Verification items for the finished model (mm, model axes). Face numbers are marked on the shaded views. A direction names the side the tool comes from. Round coordinates to 2 decimals unless told otherwise and drop trailing zeros. Write each loop counter-clockwise with the first axis right and the second up, starting at its lowest first coordinate (ties: lowest second). Pieces come first, ordered by that corner, then holes.
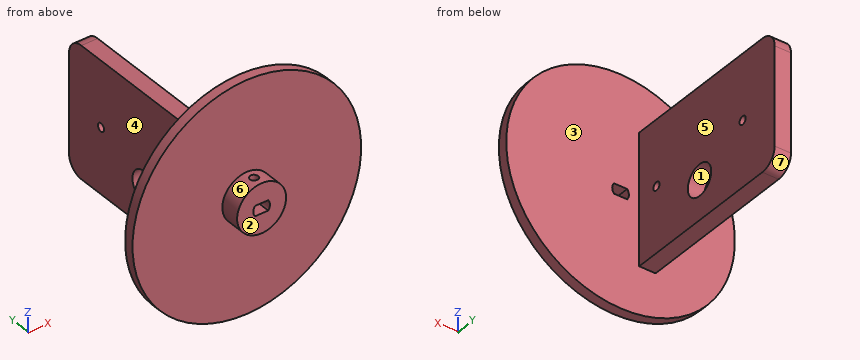
from build123d import *

# Parameters (mm, degrees)
CROQUIS1_R              = 35
SALIENTE_EXTRUIR1_DEPTH = 3
SALIENTE_EXTRUIR2_START = 6
CROQUIS2_R              = 7.5
SALIENTE_EXTRUIR2_DEPTH = 6
CROQUIS3_R              = 1.25
CORTAR_EXTRUIR1_DEPTH   = 6
CROQUIS4_W              = 5
CROQUIS4_H              = 40
SALIENTE_EXTRUIR3_DEPTH = 55
CROQUIS5_R              = 1.25
CROQUIS5_R_2            = 4.75
CORTAR_EXTRUIR2_DEPTH   = 5
REDONDEO1_R             = 5


with BuildPart() as part:
    # Croquis1 → Saliente-Extruir1 (new body)
    with BuildSketch(Plane(origin=(0, 0, 0), x_dir=(1, 0, 0), z_dir=(0, 1, 0))):
        with Locations(Location((0, 0, 0), (0, 0, 270))):
            Circle(CROQUIS1_R)
        with BuildLine():
            Line((-2.024845673, 1.55), (2.024845673, 1.55))
            ThreePointArc((2.024845673, 1.55), (2.55, 0), (2.024845673, -1.55))
            Line((2.024845673, -1.55), (-2.024845673, -1.55))
            ThreePointArc((-2.024845673, -1.55), (-2.55, 0), (-2.024845673, 1.55))
        make_face(mode=Mode.SUBTRACT)
    extrude(amount=SALIENTE_EXTRUIR1_DEPTH)

    # Croquis2 → Saliente-Extruir2 (add)
    with BuildSketch(Plane.XZ.offset(SALIENTE_EXTRUIR2_START)):
        with Locations(Location((0, 0, 0), (0, 0, 90))):
            Circle(CROQUIS2_R)
        with BuildLine():
            Line((-2.024845673, 1.55), (2.024845673, 1.55))
            ThreePointArc((2.024845673, 1.55), (2.55, 0), (2.024845673, -1.55))
            Line((2.024845673, -1.55), (-2.024845673, -1.55))
            ThreePointArc((-2.024845673, -1.55), (-2.55, 0), (-2.024845673, 1.55))
        make_face(mode=Mode.SUBTRACT)
    extrude(amount=-SALIENTE_EXTRUIR2_DEPTH)

    # Croquis3 → Cortar-Extruir1 (cut)
    with BuildSketch(Plane(origin=(0, 0, 1.55), x_dir=(-1, 0, 0), z_dir=(0, 0, -1))):
        with Locations((0, -3)):
            Circle(CROQUIS3_R)
    extrude(amount=-CORTAR_EXTRUIR1_DEPTH, mode=Mode.SUBTRACT)

    # Croquis4 → Saliente-Extruir3 (add)
    with BuildSketch(Plane(origin=(0, 3, 0), x_dir=(1, 0, 0), z_dir=(0, 1, 0))):
        with Locations((-8.215048019, 0)):
            Rectangle(CROQUIS4_W, CROQUIS4_H)
    extrude(amount=SALIENTE_EXTRUIR3_DEPTH)

    # Croquis5 → Cortar-Extruir2 (cut)
    with BuildSketch(Plane.ZY.offset(10.715048019)):
        with Locations((0, 45)):
            Circle(CROQUIS5_R)
        with Locations((0, 10)):
            Circle(CROQUIS5_R)
        with Locations((-8, 27.5)):
            Circle(CROQUIS5_R_2)
    extrude(amount=-CORTAR_EXTRUIR2_DEPTH, mode=Mode.SUBTRACT)

    # Redondeo1
    redondeo1_edges = [part.edges().sort_by_distance(p)[0] for p in [
        (-8.215048019, 58, -20),
        (-8.215048019, 58, 20),
    ]]
    fillet(redondeo1_edges, radius=REDONDEO1_R)


solid = part.part
Q1. Material ranges on line 1 along Y through (x, z) = (-6, 0); line 2 along X through (y, z) = (17, 17); line 3 along Y through (x, z) = (17.5, 18), recorded low to high.
Recorded:
line 1: y = -6 to 8.75, 11.25 to 43.75, 46.25 to 58
line 2: x = -10.72 to -5.72
line 3: y = 0 to 3
Q2. Sectioned sample at D-D (y = -3). Enter the section's corners in (x, z).
Recorded:
outline: (-2.02, -1.55) arc R2.55 cw to (-2.02, 1.55) - (-1.25, 1.55) - (-1.25, 7.4) arc R7.5 ccw (long way) to (1.25, 7.4) - (1.25, 1.55) - (2.02, 1.55) arc R2.55 cw to (2.02, -1.55) - close
Q3. Sectioned sample at B-B (y = 45). Enter the section's corners in (x, z).
Recorded:
outline: (-10.72, -20) - (-5.72, -20) - (-5.72, -1.25) - (-10.72, -1.25) - close; (-10.72, 1.25) - (-5.72, 1.25) - (-5.72, 20) - (-10.72, 20) - close
Q4. Sectioned sample at A-A (z = 0). Enter the section's corners in (x, y).
Recorded:
outline: (-35, 0) - (-7.5, 0) - (-7.5, -6) - (-2.55, -6) - (-2.55, 3) - (-5.72, 3) - (-5.72, 8.75) - (-10.72, 8.75) - (-10.72, 3) - (-35, 3) - close; (-10.72, 11.25) - (-5.72, 11.25) - (-5.72, 43.75) - (-10.72, 43.75) - close; (-10.72, 46.25) - (-5.72, 46.25) - (-5.72, 58) - (-10.72, 58) - close; (2.55, -6) - (7.5, -6) - (7.5, 0) - (35, 0) - (35, 3) - (2.55, 3) - close
Q5. Depth check by flat-ended pin: P1, Ø12, axis at y = 50, z = -24, coming from the +X side; P2, Ø4, axis at x = -13, y = 3.5, coming from the -Z side; P3, Ø1.5, axis at x = 16, z = 6, coming from the -Y side. Enter the tip coordinate at first touch or a pass-through.
Recorded:
P1: stops at x = -5.72
P2: stops at z = -33.21
P3: stops at y = 0
Q6. Tool access check on the marked faces 5, 6 and 7. Record the directions out of +Z, -Z, +X, -X, +Y, -Y that give a thin tool (end or side, any length) a straight path to the whole face; none if there is none.
Recorded:
face 5: +Z, -Z, +X, +Y
face 6: -Y
face 7: -Z, +X, -X, +Y
Q7. Sectioned sample at C-C (z = -17.5). Enter the section's corners in (x, y), plus the area to 3 significant figures.
Recorded:
outline: (-30.31, 0) - (30.31, 0) - (30.31, 3) - (-5.72, 3) - (-5.72, 57.33) - (-10.72, 57.33) - (-10.72, 3) - (-30.31, 3) - close
area: 454 mm2
Q8. Release check for a two-part mould opening along Y. For the marked faces 1, 2, 3 and 4 record: released by +Y, released by -Y, zero draft, split by the parting line, or undercut.
Recorded:
face 1: undercut
face 2: released by -Y
face 3: released by +Y
face 4: zero draft
